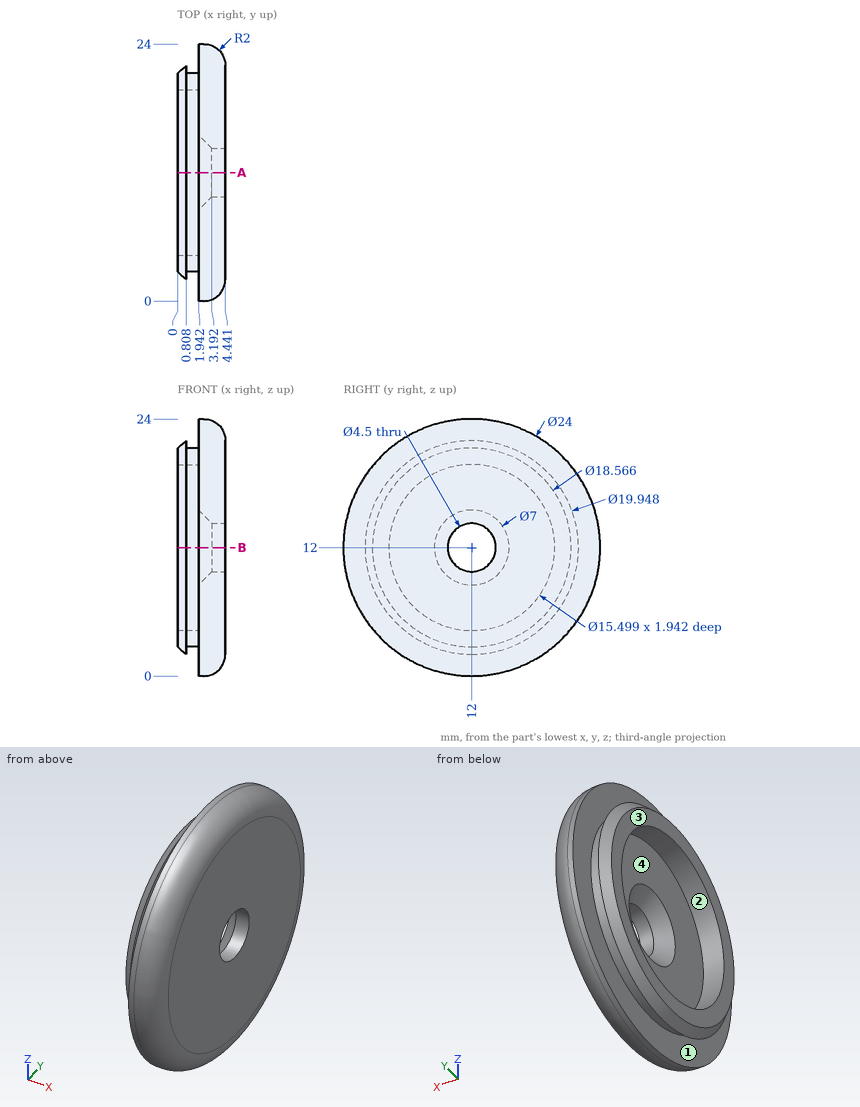
Job drawing, mm, ordinate dimensions from the low corner. One solid piece. A direction names the side the tool comes from. Give positions to 0.01 mm unless a question says otherwise; leave off trailing zeros. Loops run counter-clockwise (first coordinate to the right, second up) from the corner with the lowest first, then second, coordinate; pieces in that order, holes last. Notation, with made-up numbers: M 45.25,60 L 55.25,60 A30 cw 55.25,82 Z; hole C -2,7.25 d6. An arc over 180 degrees is marked long. Answer in a Markdown table with one row per item. Add a question column.
Item 1: Drop flat-ended pins along their axis: P1, Ø3.5, axis at y = 12, z = 12, coming from the +X side; P2, Ø12.5, axis at y = 13.5, z = 10, coming from the -X side; P3, Ø2, axis at x = 3.5, z = 11.5, coming from the -Y side (1 decimal); P4, Ø9.5, axis at y = 12, z = 12, coming from the -X side. Give the stop position or say it passes through.
Item 2: Tool access for the marked faces 3 and 4: list every direction of +Z, -Z, +X, -X, +Y, -Y with a clear straight run to the whole face (end or side of a thin tool).
Item 3: Band-saw the part on A-A on y = 12. Give the cut face in (x, z).
Item 4: Probe probe 1 along Y at (x, z) = (0.85, 12); probe 2 along Y at (x, z) = (3.9, 12); probe 3 along X at (y, z) = (14, 8.75). List the from-to ranges inside material, lowest first.
Item 5: Mould opens along Y. For the marked faces 1 and 2 say: +Y half, -Y half, draft (parallel to the pull), parting line (faces both ways), or undercut.
Reply:
| question | item | result |
|---|---|---|
| 1 | P1 | passes through |
| 1 | P2 | stops at x = 0 |
| 1 | P3 | stops at y = 0 |
| 1 | P4 | stops at x = 1.94 |
| 2 | face 3 | +Z, -Z, -X, +Y, -Y |
| 2 | face 4 | -X |
| 3 | outline | M 0,2.72 L 0.81,2.03 L 0.81,2.72 L 1.94,2.72 L 1.94,0 L 2.44,0 A2 ccw 4.44,2 L 4.44,9.75 L 3.19,9.75 L 1.94,8.5 L 1.94,4.25 L 0,4.25 Z; M 0,19.75 L 1.94,19.75 L 1.94,15.5 L 3.19,14.25 L 4.44,14.25 L 4.44,22 A2 ccw 2.44,24 L 1.94,24 L 1.94,21.28 L 0.81,21.28 L 0.81,21.97 L 0,21.28 Z |
| 4 | probe 1 | y = 2.72 to 4.25, 19.75 to 21.28 |
| 4 | probe 2 | y = 0.63 to 9.75, 14.25 to 23.37 |
| 4 | probe 3 | x = 1.94 to 4.44 |
| 5 | face 1 | draft |
| 5 | face 2 | undercut |
